Geometry: see drawing. Coordinates: mm, zero at the bounding-box minimum. A direction names the side the tool comes from. Coordinates: 2 decimals unless noted, no trailing zeros. Loops run counter-clockwise (first coordinate to the right, second up) from the corner with the lowest first, then second, coordinate; pieces in that order, holes last.
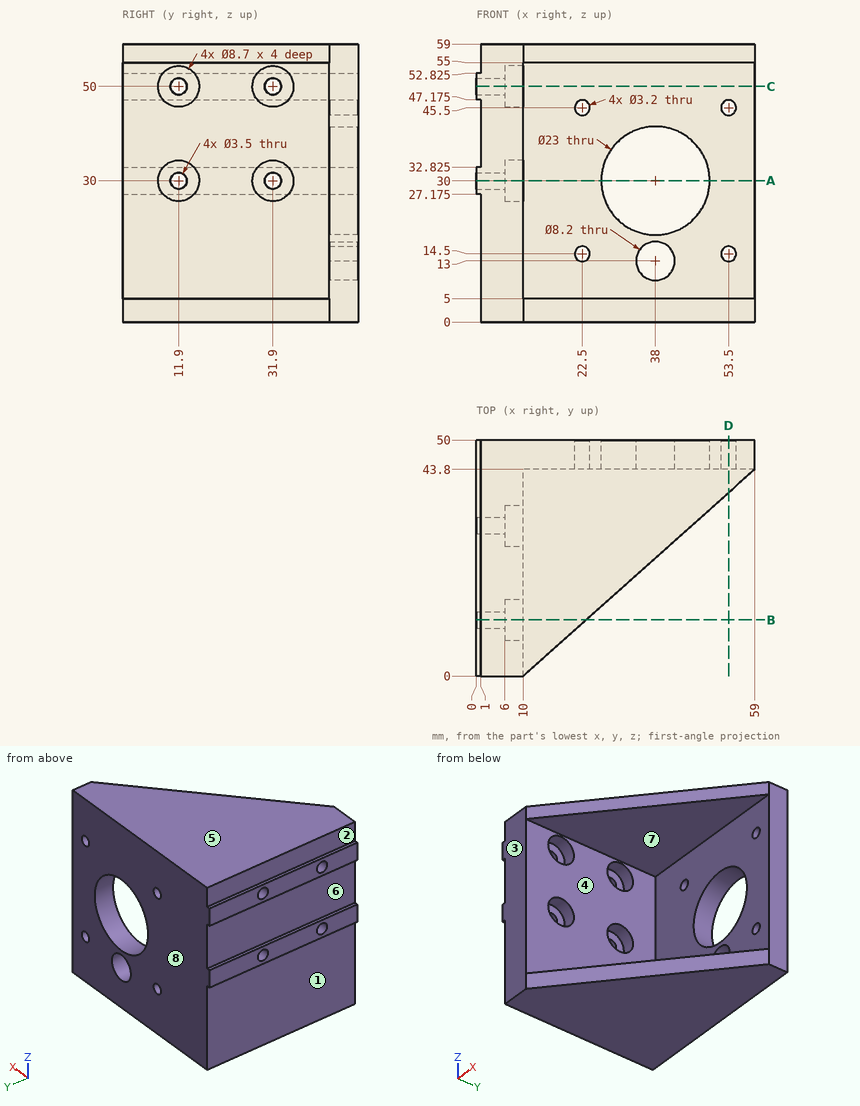
Item 1: Reachability of the marked faces 1, 2, 3 and 4 from +Z, -Z, +X, -X, +Y, -Y: full face, straight path, thin tool, end or side. Return the list, or none.
Result:
face 1: -Z, -X, +Y, -Y
face 2: +Z, -X, +Y, -Y
face 3: +Z, -Z, +X, -X, -Y
face 4: +X, -Y
Item 2: Section query D-D (x = 53.5). Output: boundary loops of the cut face in (y, z).
Result:
outline: (38.88, 0) - (50, 0) - (50, 12.9) - (43.8, 12.9) - (43.8, 5) - (38.88, 5) - close; (38.88, 55) - (43.8, 55) - (43.8, 47.1) - (50, 47.1) - (50, 59) - (38.88, 59) - close; (43.8, 16.1) - (50, 16.1) - (50, 43.9) - (43.8, 43.9) - close
Item 3: Mould query, pull axis Z, two halves, no side actions, for the marked faces 5, 6, 7 and 8. Classes: +Z half, -Z half, draft (parallel to the pull), parting line (faces both ways), or undercut.
Result:
face 5: +Z half
face 6: undercut
face 7: undercut
face 8: draft
Item 4: Line query: L1, parallel to Y at x = 4, z = 50; L2, parallel to Z at x = 3.25, y = 31.9; L3, parallel to Z at x = 36, y = 25. Output: solid intervals per line, ascending.
Result:
L1: y = 0 to 10.15, 13.65 to 30.15, 33.65 to 50
L2: z = 0 to 28.25, 31.75 to 48.25, 51.75 to 59
L3: z = 0 to 5, 55 to 59
Item 5: Contact query for flat-ended pins moving along their axis: P1, Ø1.1, axis at x = 0.5, y = 23, coming from the +Z side; P2, Ø1, axis at x = 44, z = 48, coming from the -Y side; P3, Ø3, axis at x = 22.5, z = 14.5, coming from the -Y side (3 decimals); P4, Ø7, axis at y = 34, z = 48, coming from the +X side. Output: stop coordinate, or through.
Result:
P1: stops at z = 59
P2: stops at y = 43.8
P3: passes through
P4: stops at x = 10
Item 6: Section query C-C (z = 50). Output: boundary loops of the cut face in (x, y), then the cut area to 3 significant figures.
Result:
outline: (0, 0) - (10, 0) - (10, 7.55) - (6, 7.55) - (6, 10.15) - (0, 10.15) - close; (0, 13.65) - (6, 13.65) - (6, 16.25) - (10, 16.25) - (10, 27.55) - (6, 27.55) - (6, 30.15) - (0, 30.15) - close; (0, 33.65) - (6, 33.65) - (6, 36.25) - (10, 36.25) - (10, 43.8) - (59, 43.8) - (59, 50) - (0, 50) - close
area: 692 mm2
Item 7: Section query B-B (y = 11.9). Count the separate pieces of the cut face and the enclosed holes in it, then the cut area to 3 significant figures.
Result:
separate pieces: 3
enclosed holes: 0
area: 551 mm2
Item 8: Section query A-A (z = 30). Output: boundary loops of the cut face in (x, y), then the cut area to 3 significant figures.
Result:
outline: (0, 0) - (10, 0) - (10, 7.55) - (6, 7.55) - (6, 10.15) - (0, 10.15) - close; (0, 13.65) - (6, 13.65) - (6, 16.25) - (10, 16.25) - (10, 27.55) - (6, 27.55) - (6, 30.15) - (0, 30.15) - close; (0, 33.65) - (6, 33.65) - (6, 36.25) - (10, 36.25) - (10, 43.8) - (26.5, 43.8) - (26.5, 50) - (0, 50) - close; (49.5, 43.8) - (59, 43.8) - (59, 50) - (49.5, 50) - close
area: 550 mm2
